```python
from build123d import *

# Parameters (mm, degrees)
SKETCH1_W                  = 18.669
SKETCH1_H                  = 69.469
BOSS_EXTRUDE1_DEPTH        = 12.192
TAP_DRILL_FOR_10_32_TAP1_D = 4.0386
TAP_DRILL_FOR_10_32_TAP2_D = 4.0386


with BuildPart() as part:
    # Sketch1 → Boss-Extrude1 (new body)
    with BuildSketch(Plane.XY):
        Rectangle(SKETCH1_W, SKETCH1_H)
    extrude(amount=BOSS_EXTRUDE1_DEPTH)

    # Tap Drill for #10-32 Tap1 (through all)
    with Locations(Plane(origin=(9.3345, 0, 0), x_dir=(0, 0, -1), z_dir=(1, 0, 0))):
        with Locations((-6.096, 19.05), (-6.096, -19.05)):
            Hole(TAP_DRILL_FOR_10_32_TAP1_D / 2)

    # Tap Drill for #10-32 Tap2 (through all)
    with Locations(Plane.XY.offset(12.192)):
        with Locations((0, 27.94), (0, -27.94), (0, 0)):
            Hole(TAP_DRILL_FOR_10_32_TAP2_D / 2)


solid = part.part
```
For this review, take the finished solid that the model builds, in its own axes (mm). Coordinates: 2 decimals unless noted, no trailing zeros. Loops run counter-clockwise (first coordinate to the right, second up) from the corner with the lowest first, then second, coordinate; pieces in that order, holes last.
1. Add section B-B, the plane x = 2.75. Give the boundary of the cut face in (y, z), then the cut area to 3 significant figures.
2. Add section C-C, the plane z = 7. Give the boundary of the cut face in (x, y), then the cut area to 3 significant figures.
3. Insertion check: P1, Ø3, axis at x = 0, y = -27.94, coming from the +Z side. The pin has a flat end and moves straight along its axis. Give the tip position at first contact, or say it passes through.
4. Add section D-D, the plane z = 11.25. Give the boundary of the cut face in (x, y), then the cut area to 3 significant figures.
5. Mouldability with a two-part tool opening along Z and no side actions: class faces 1 (the cylindrical face through (-0.13, -17.05, 5.83)), 2 (the flat face through (-2.2, 0.5, 0)), 3 (the flat face through (0, -34.734, 6)) as +Z half, -Z half, draft (parallel to the pull), parting line (faces both ways), or undercut.
6. Add section A-A, the plane y = 19.05. Give the boundary of the cut face in (x, z).
7. For line 1 (Y direction, x = 0, z = 4); line 2 (Y direction, x = -1, z = 8.25); line 3 (Y direction, x = 0, z = 6.25), list the stretches that pass through material, from the lowest coordinate up.
Result:
1. outline: (-34.73, 0) - (34.73, 0) - (34.73, 12.19) - (-34.73, 12.19) - close; hole circle Ø4.04 at (-19.05, 6.1); hole circle Ø4.04 at (19.05, 6.1)
1. area: 821 mm2
2. outline: (-9.33, -34.73) - (9.33, -34.73) - (9.33, -20.86) - (-9.33, -20.86) - close; (-9.33, -17.24) - (9.33, -17.24) - (9.33, 17.24) - (-9.33, 17.24) - close; (-9.33, 20.86) - (9.33, 20.86) - (9.33, 34.73) - (-9.33, 34.73) - close; hole circle Ø4.04 at (0, -27.94); hole circle Ø4.04 at (0, 0); hole circle Ø4.04 at (0, 27.94)
2. area: 1,120 mm2
3. P1: passes through
4. outline: (-9.33, -34.73) - (9.33, -34.73) - (9.33, 34.73) - (-9.33, 34.73) - close; hole circle Ø4.04 at (0, -27.94); hole circle Ø4.04 at (0, 0); hole circle Ø4.04 at (0, 27.94)
4. area: 1,260 mm2
5. face 1: undercut
5. face 2: -Z half
5. face 3: draft
6. outline: (-9.33, 0) - (9.33, 0) - (9.33, 4.08) - (-9.33, 4.08) - close; (-9.33, 8.12) - (9.33, 8.12) - (9.33, 12.19) - (-9.33, 12.19) - close
7. line 1: y = -34.73 to -29.96, -25.92 to -2.02, 2.02 to 25.92, 29.96 to 34.73
7. line 2: y = -34.73 to -29.69, -26.19 to -1.75, 1.75 to 26.19, 29.69 to 34.73
7. line 3: y = -34.73 to -29.96, -25.92 to -21.06, -17.04 to -2.02, 2.02 to 17.04, 21.06 to 25.92, 29.96 to 34.73
